```python
from build123d import *

# Parameters (mm, degrees)
F1_DEPTH = 3
F3_D     = 3
F5_D     = 3
F7_D     = 3
F9_D     = 15


with BuildPart() as f1:
    # F0 (on Top) → F1 (new body)
    with BuildSketch(Plane.XY):
        with BuildLine():
            Line((-25, 80.777472107), (-75, 80.777472107))
            ThreePointArc((-75, 80.777472107), (-120, 0), (-75, -80.777472107))
            Line((-75, -80.777472107), (-25, -80.777472107))
            ThreePointArc((-25, -80.777472107), (-70, 0), (-25, 80.777472107))
        make_face()
        with BuildLine():
            Line((25, 80.777472107), (-25, 80.777472107))
            ThreePointArc((-25, 80.777472107), (-70, 0), (-25, -80.777472107))
            Line((-25, -80.777472107), (25, -80.777472107))
            ThreePointArc((25, -80.777472107), (57.9909633635, -46.2331050223), (70, 0))
            ThreePointArc((70, 0), (57.9909633635, 46.2331050223), (25, 80.777472107))
        make_face()
        with BuildLine():
            Line((75, 80.777472107), (25, 80.777472107))
            ThreePointArc((25, 80.777472107), (57.9909633635, 46.2331050223), (70, 0))
            ThreePointArc((70, 0), (57.9909633635, -46.2331050223), (25, -80.777472107))
            Line((25, -80.777472107), (75, -80.777472107))
            ThreePointArc((75, -80.777472107), (107.9909633635, -46.2331050223), (120, 0))
            ThreePointArc((120, 0), (107.9909633635, 46.2331050223), (75, 80.777472107))
        make_face()
    extrude(amount=F1_DEPTH)

    # F3 (through all)
    with Locations(Plane.XY.offset(3)):
        with Locations((-50, 50), (50, 50), (50, -50), (-50, -50)):
            Hole(F3_D / 2)

    # F5 (through all)
    with Locations(Plane.XY.offset(3)):
        with Locations((-21.2132034356, 21.2132034356), (21.2132034356, 21.2132034356), (21.2132034356, -21.2132034356), (-21.2132034356, -21.2132034356)):
            Hole(F5_D / 2)

    # F7 (through all)
    with Locations(Plane(origin=(0, 0, 0), x_dir=(1, 0, 0), z_dir=(0, 0, -1))):
        with Locations((-24.5, 41.5), (24.5, 41.5), (24.5, -16.5), (-24.5, -16.5)):
            Hole(F7_D / 2)

    # F9 (through all)
    with Locations(Plane.XY.offset(3)):
        with Locations((-80, 0)):
            Hole(F9_D / 2)


solid = f1.part
```
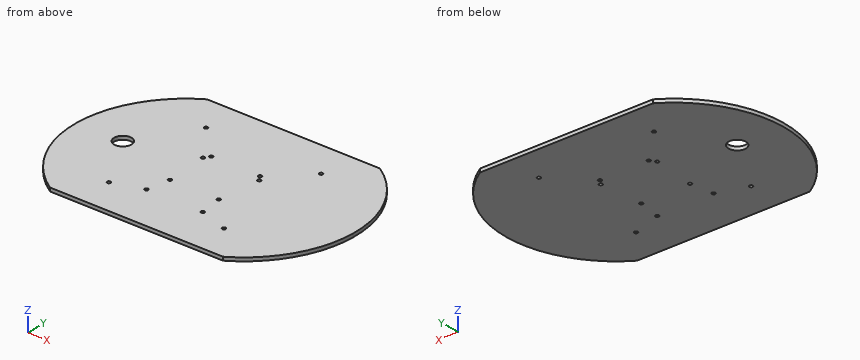
Geometry check sheet. Reference: the model listing, model coordinates, mm. Coordinates: 2 decimals unless noted, no trailing zeros. Write each loop counter-clockwise with the first axis right and the second up, starting at its lowest first coordinate (ties: lowest second). Pieces come first, ordered by that corner, then holes. Notation, with made-up numbers: M 72.25,-20 L 108.25,-20 A22 ccw 108.25,7 Z; hole C 46,62.25 d4. An arc over 180 degrees is marked long. One line per item, written item: value. Start each with the question number.
(1) Sectioned sample at B-B, the plane x = -80. Enter the section's corners in (y, z), and give its area (3 significant figures).
(2) Sectioned sample at C-C, the plane y = 3. Enter the section's corners in (x, z).
(3) Sectioned sample at D-D, the plane y = -25.5. Enter the section's corners in (x, z), and give its area (3 significant figures).
(4) Depth check by flat-ended pin: pin 1 (1.8 mm diameter, centred on x = -21.21, y = -21.21, fed in from +Z). Enter the tip coordinate at first touch or a pass-through.
(5) Sectioned sample at A-A, the plane z = 0.8. State how many separate pieces and enclosed holes the cut face has, and give its area (3 significant figures).
(6) Scan lines: line 1 along Y through (x, z) = (-24.5, 0.9); line 2 along X through (y, z) = (21.5, 0.7); line 3 along X through (y, z) = (21, 1.7). Record each from-to range of solid material in increasing order. Write a range as [from, to].
Filled sheet:
1. outline: M -77.46,0 L -7.5,0 L -7.5,3 L -77.46,3 Z; M 7.5,0 L 77.46,0 L 77.46,3 L 7.5,3 Z
1. area: 420 mm²
2. outline: M -119.95,0 L -86.87,0 L -86.87,3 L -119.95,3 Z; M -73.13,0 L 119.95,0 L 119.95,3 L -73.13,3 Z
3. outline: M -116.51,0 L 116.51,0 L 116.51,3 L -116.51,3 Z
3. area: 699 mm²
4. pin 1: through
5. separate pieces: 1
5. enclosed holes: 13
5. area: 34,200 mm²
6. line 1: [-80.78, -43], [-40, 15], [18, 80.78]
6. line 2: [-117.54, -22.69], [-19.74, 19.74], [22.69, 117.54]
6. line 3: [-117.65, -22.7], [-19.73, 19.73], [22.7, 117.65]
